from build123d import *

# Parameters (mm, degrees)
SKETCH_1_W                = 130
SKETCH_1_H                = 64
EXTRUDE_1_DEPTH           = 125
SKETCH_2_W                = 55.4
SKETCH_2_H                = 114
CUT_EXTRUDE_1_DEPTH       = 47
SKETCH_3_W                = 45.4
SKETCH_3_H                = 86
CUT_EXTRUDE_2_DEPTH       = 78
SKETCH_4_W                = 24.038907643
SKETCH_4_H                = 40
CUT_EXTRUDE_3_DEPTH       = 40
SKETCH_5_W                = 4.3
SKETCH_5_H                = 25
CUT_EXTRUDE_4_DEPTH       = 25
SKETCH_6_W                = 10
SKETCH_6_H                = 40
CUT_EXTRUDE_5_DEPTH       = 35
SKETCH_9_W                = 5
SKETCH_9_H                = 125
CUT_EXTRUDE_8_DEPTH       = 155.744951452
SKETCH_10_W               = 20
SKETCH_10_H               = 150
EXTRUDE_2_DEPTH           = 5
SKETCH_11_R               = 2.5
CUT_EXTRUDE_9_DEPTH       = 159.941026799
FILLET_1_R                = 3
SKETCH_12_W               = 32
SKETCH_12_H               = 30
CUT_EXTRUDE_10_DEPTH      = 161.864073055
SKETCH_13_W               = 45
SKETCH_13_H               = 50
CUT_EXTRUDE_11_DEPTH      = 30
FILLET_5_R                = 5
SKETCH_14_W               = 32
SKETCH_14_H               = 150
CUT_EXTRUDE_12_DEPTH      = 185.946613919
SKETCH_16_W               = 14.899109585
SKETCH_16_H               = 40
CUT_EXTRUDE_14_DEPTH      = 40
CUT_EXTRUDE_15_DEPTH      = 143.707007536
CUT_EXTRUDE_15_DEPTH_BACK = 143.707007536
SKETCH_17_W               = 30
SKETCH_17_H               = 95
SKETCH_18_W               = 20
SKETCH_18_H               = 6
CUT_EXTRUDE_16_DEPTH      = 150.244765402
SKETCH_20_W               = 47
SKETCH_20_H               = 10
EXTRUDE_3_DEPTH           = 10
SKETCH_21_R               = 1.75
CUT_EXTRUDE_17_DEPTH      = 141.388745988
SKETCH_23_W               = 42
SKETCH_23_H               = 27.7
CUT_EXTRUDE_19_DEPTH      = 138.927517197
EXTRUDE_4_DEPTH           = 27.7
SKETCH_25_W               = 48
SKETCH_25_H               = 23
EXTRUDE_5_DEPTH           = 4.3
FILLET_6_R                = 5
FILLET_8_R                = 5
CUT_EXTRUDE_23_DEPTH      = 10
SKETCH_31_R               = 1.55
CUT_EXTRUDE_24_DEPTH      = 138.669895039
FILLET_9_R                = 5
FILLET_10_R               = 5
FILLET_11_R               = 5


with BuildPart() as part:
    # 草图1 → 凸台-拉伸1 (new body)
    with BuildSketch(Plane(origin=(0, 0, 0), x_dir=(1, 0, 0), z_dir=(0, 1, 0))):
        Rectangle(SKETCH_1_W, SKETCH_1_H)
    extrude(amount=EXTRUDE_1_DEPTH)

    # 草图2 → 切除-拉伸1 (cut)
    with BuildSketch(Plane(origin=(65, 0, 0), x_dir=(0, 0, -1), z_dir=(1, 0, 0))):
        with Locations((0, 62)):
            Rectangle(SKETCH_2_W, SKETCH_2_H)
    extrude(amount=-CUT_EXTRUDE_1_DEPTH, mode=Mode.SUBTRACT)

    # 草图3 → 切除-拉伸2 (cut)
    with BuildSketch(Plane(origin=(18, 0, 0), x_dir=(0, 0, -1), z_dir=(1, 0, 0))):
        with Locations((0, 48)):
            Rectangle(SKETCH_3_W, SKETCH_3_H)
    extrude(amount=-CUT_EXTRUDE_2_DEPTH, mode=Mode.SUBTRACT)

    # 草图4 → 切除-拉伸3 (cut)
    with BuildSketch(Plane(origin=(65, 0, 0), x_dir=(0, 0, -1), z_dir=(1, 0, 0))):
        with Locations((26.569318974, 55)):
            Rectangle(SKETCH_4_W, SKETCH_4_H)
    extrude(amount=-CUT_EXTRUDE_3_DEPTH, mode=Mode.SUBTRACT)

    # 草图5 → 切除-拉伸4 (cut)
    with BuildSketch(Plane(origin=(65, 0, 0), x_dir=(0, 0, -1), z_dir=(1, 0, 0))):
        with Locations((29.85, 87.5)):
            Rectangle(SKETCH_5_W, SKETCH_5_H)
    extrude(amount=-CUT_EXTRUDE_4_DEPTH, mode=Mode.SUBTRACT)

    # 草图6 → 切除-拉伸5 (cut)
    with BuildSketch(Plane(origin=(0, 125, 0), x_dir=(1, 0, 0), z_dir=(0, 1, 0))):
        with Locations((45, 0)):
            Rectangle(SKETCH_6_W, SKETCH_6_H)
    extrude(amount=-CUT_EXTRUDE_5_DEPTH, mode=Mode.SUBTRACT)

    # 草图9 → 切除-拉伸8 (cut, through all)
    with BuildSketch(Plane.XY.offset(32)):
        with Locations((62.5, 62.5)):
            Rectangle(SKETCH_9_W, SKETCH_9_H)
    extrude(amount=-CUT_EXTRUDE_8_DEPTH, mode=Mode.SUBTRACT)

    # 草图10 → 凸台-拉伸2 (add)
    with BuildSketch(Plane(origin=(0, 0, -32), x_dir=(-1, 0, 0), z_dir=(0, 0, -1))):
        with Locations((15, 57.5)):
            Rectangle(SKETCH_10_W, SKETCH_10_H)
    extrude(amount=-EXTRUDE_2_DEPTH)

    # 草图11 → 切除-拉伸9 (cut, through all)
    with BuildSketch(Plane.XY.offset(-27)):
        with Locations((-15, -12)):
            Circle(SKETCH_11_R)
        with Locations((-15, 137)):
            Circle(SKETCH_11_R)
    extrude(amount=-CUT_EXTRUDE_9_DEPTH, mode=Mode.SUBTRACT)

    # 圆角1
    fillet_1_edges = [part.edges().sort_by_distance(p)[0] for p in [
        (-15, 0, -27),
        (-5, 0, -29.5),
        (-25, 0, -29.5),
        (-25, 132.5, -29.5),
        (-25, 125, -29.5),
        (-5, 125, -29.5),
        (-15, 125, -27),
        (-25, -17.5, -29.5),
        (-5, -17.5, -29.5),
        (-5, 132.5, -29.5),
    ]]
    fillet(fillet_1_edges, radius=FILLET_1_R)

    # 草图12 → 切除-拉伸10 (cut, through all)
    with BuildSketch(Plane.XY.offset(32)):
        with Locations((-49, 110)):
            Rectangle(SKETCH_12_W, SKETCH_12_H)
    extrude(amount=-CUT_EXTRUDE_10_DEPTH, mode=Mode.SUBTRACT)

    # 草图13 → 切除-拉伸11 (cut)
    with BuildSketch(Plane(origin=(0, 125, 0), x_dir=(1, 0, 0), z_dir=(0, 1, 0))):
        with Locations((-10.5, -7)):
            Rectangle(SKETCH_13_W, SKETCH_13_H)
    extrude(amount=-CUT_EXTRUDE_11_DEPTH, mode=Mode.SUBTRACT)

    # 圆角5
    fillet_5_edges = [part.edges().sort_by_distance(p)[0] for p in [
        (-33, 110, -18),
        (12, 110, -18),
    ]]
    fillet(fillet_5_edges, radius=FILLET_5_R)

    # 草图14 → 切除-拉伸12 (cut, through all)
    with BuildSketch(Plane.ZY.offset(65)):
        with Locations((-16, 57.5)):
            Rectangle(SKETCH_14_W, SKETCH_14_H)
    extrude(amount=-CUT_EXTRUDE_12_DEPTH, mode=Mode.SUBTRACT)

    # 草图16 → 切除-拉伸14 (cut)
    with BuildSketch(Plane(origin=(60, 0, 0), x_dir=(0, 0, -1), z_dir=(1, 0, 0))):
        with Locations((-29.056746571, 55)):
            Rectangle(SKETCH_16_W, SKETCH_16_H)
    extrude(amount=-CUT_EXTRUDE_14_DEPTH, mode=Mode.SUBTRACT)

    # 草图17 → 切除-拉伸15 (cut, two sides: drawn at the far end of the back side and taken through both)
    with BuildSketch(Plane(origin=(0, 0, 22.7), x_dir=(-1, 0, 0), z_dir=(0, 0, -1)).offset(-CUT_EXTRUDE_15_DEPTH_BACK)):
        with Locations((50, 47.5)):
            Rectangle(SKETCH_17_W, SKETCH_17_H)
    extrude(amount=CUT_EXTRUDE_15_DEPTH + CUT_EXTRUDE_15_DEPTH_BACK, mode=Mode.SUBTRACT)

    # 草图18 → 切除-拉伸16 (cut, through all)
    with BuildSketch(Plane(origin=(40, 0, 0), x_dir=(0, 0, -1), z_dir=(1, 0, 0))):
        with Locations((-10, 122)):
            Rectangle(SKETCH_18_W, SKETCH_18_H)
    extrude(amount=CUT_EXTRUDE_16_DEPTH, mode=Mode.SUBTRACT)

    # 草图20 → 凸台-拉伸3 (add)
    with BuildSketch(Plane.XY.offset(32)):
        with Locations((-11.5, -5)):
            Rectangle(SKETCH_20_W, SKETCH_20_H)
        with Locations((-11.5, 100)):
            Rectangle(SKETCH_20_W, SKETCH_20_H)
    extrude(amount=-EXTRUDE_3_DEPTH)

    # 草图21 → 切除-拉伸17 (cut, through all)
    with BuildSketch(Plane(origin=(0, 0, 22), x_dir=(-1, 0, 0), z_dir=(0, 0, -1))):
        with Locations(Location((25, -5, 0), (0, 0, 180))):
            Circle(SKETCH_21_R)
        with Locations(Location((5, -5, 0), (0, 0, 180))):
            Circle(SKETCH_21_R)
        with Locations((5, 100)):
            Circle(SKETCH_21_R)
        with Locations((25, 100)):
            Circle(SKETCH_21_R)
    extrude(amount=-CUT_EXTRUDE_17_DEPTH, mode=Mode.SUBTRACT)

    # 草图23 → 切除-拉伸19 (cut, through all)
    with BuildSketch(Plane(origin=(0, 5, 0), x_dir=(1, 0, 0), z_dir=(0, 1, 0))):
        with Locations((39, -13.85)):
            Rectangle(SKETCH_23_W, SKETCH_23_H)
    extrude(amount=-CUT_EXTRUDE_19_DEPTH, mode=Mode.SUBTRACT)

    # 草图24 → 凸台-拉伸4 (add)
    with BuildSketch(Plane(origin=(0, 0, 0), x_dir=(-1, 0, 0), z_dir=(0, 0, -1))):
        Polygon((-18, 0), (-18, -17), (-60, -17), (-60, -23), (-12, -23), (-12, 0), align=None)
    extrude(amount=-EXTRUDE_4_DEPTH)

    # 草图25 → 凸台-拉伸5 (add)
    with BuildSketch(Plane.XY.offset(32)):
        with Locations((36, -11.5)):
            Rectangle(SKETCH_25_W, SKETCH_25_H)
    extrude(amount=-EXTRUDE_5_DEPTH)

    # 圆角6
    fillet_6_edges = [part.edges().sort_by_distance(p)[0] for p in [
        (-35, 105, 27),
        (12, 105, 27),
        (-35, -10, 27),
        (12, -10, 27),
    ]]
    fillet(fillet_6_edges, radius=FILLET_6_R)

    # 圆角8
    fillet_8_edges = [part.edges().sort_by_distance(p)[0] for p in [
        (12, 95, 11),
    ]]
    fillet(fillet_8_edges, radius=FILLET_8_R)

    # 草图30 → 切除-拉伸23 (cut)
    with BuildSketch(Plane(origin=(0, 0, 22), x_dir=(-1, 0, 0), z_dir=(0, 0, -1))):
        with BuildLine():
            Line((-7, 105), (-3, 105))
            Line((-3, 105), (-3, 95))
            Line((-3, 95), (-7, 95))
            ThreePointArc((-7, 95), (-10.535533906, 96.464466094), (-12, 100))
            Line((-12, 100), (-12, 110))
            ThreePointArc((-12, 110), (-10.535533906, 106.464466094), (-7, 105))
        make_face()
        with BuildLine():
            Line((-7, -10), (-3, -10))
            Line((-3, -10), (-3, 0))
            Line((-3, 0), (-12, 0))
            Line((-12, 0), (-12, -15))
            ThreePointArc((-12, -15), (-10.535533906, -11.464466094), (-7, -10))
        make_face()
    extrude(amount=-CUT_EXTRUDE_23_DEPTH, mode=Mode.SUBTRACT)

    # 草图31 → 切除-拉伸24 (cut, through all)
    with BuildSketch(Plane.ZY.offset(-12)):
        with Locations(Location((23.7, 113.3, 0), (0, 0, 270))):
            Circle(SKETCH_31_R)
        with Locations(Location((23.7, -12.3, 0), (0, 0, 270))):
            Circle(SKETCH_31_R)
    extrude(amount=-CUT_EXTRUDE_24_DEPTH, mode=Mode.SUBTRACT)

    # 圆角9
    fillet_9_edges = [part.edges().sort_by_distance(p)[0] for p in [
        (12, 0, 16),
    ]]
    fillet(fillet_9_edges, radius=FILLET_9_R)

    # 圆角10
    fillet_10_edges = [part.edges().sort_by_distance(p)[0] for p in [
        (3, -10, 27),
    ]]
    fillet(fillet_10_edges, radius=FILLET_10_R)

    # 圆角11
    fillet_11_edges = [part.edges().sort_by_distance(p)[0] for p in [
        (3, 105, 27),
    ]]
    fillet(fillet_11_edges, radius=FILLET_11_R)


solid = part.part
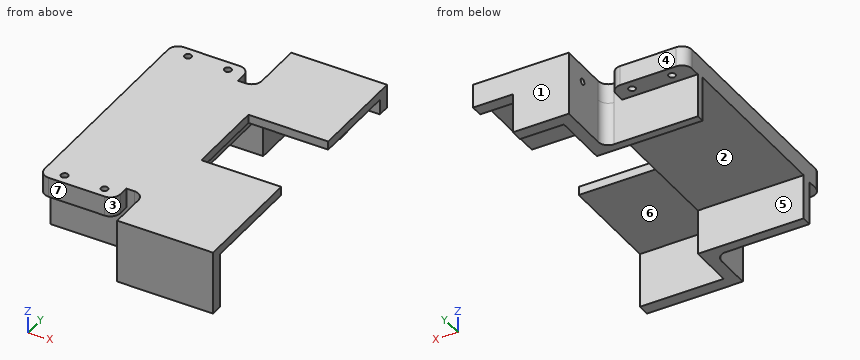
Work out the finished part from the listing and answer in its coordinate system (mm). Face numbers are marked on the shaded views. A direction names the side the tool comes from. Coordinates: 2 decimals unless noted, no trailing zeros. Write each loop counter-clockwise with the first axis right and the second up, starting at its lowest first coordinate (ties: lowest second). Pieces come first, ordered by that corner, then holes. Notation, with made-up numbers: M 80,-35 L 84,-35 A13 ccw 84,-21 Z; hole C -3.5,23.5 d7. An arc over 180 degrees is marked long. Write item = value, one per line.
1. Flat-ended cylindrical pins translate along their axes: pin 1 (8 mm diameter, centred on x = 5.5, z = 17.5, fed in from +Y); pin 2 (1.3 mm diameter, centred on y = 57.5, z = 29.5, fed in from +X); pin 3 (14 mm diameter, centred on y = 75, z = 20.5, fed in from +X). Find the tip coordinate at first contact, or state that the pin passes through.
Solution:
pin_1 = 95.67
pin_2 = 20
pin_3 = 18
2. Determine the mould class of the marked faces 1, 2 and 3 for opening direction Y: released by +Y, released by -Y, zero draft, split by the parting line, or undercut.
Solution:
face_1 = released by +Y
face_2 = undercut
face_3 = released by -Y
3. The part is cut by section B-B (x = 46.5). Determine the outline of the cut face in (y, z).
Solution:
outline = M -23,0 L -17,0 L -17,27.7 L 35,27.7 L 35,32 L -23,32 Z; M 75,27.7 L 119,27.7 L 119,20 L 125,20 L 125,32 L 75,32 Z
4. Straight lines are drawn through the part: line 1 (X direction, y = 100, z = 24.5); line 2 (X direction, y = 100, z = 30.25); line 3 (Y direction, x = -25, z = 24). For each, find the intervals that lie inside material, in ascending order. Write a range as from..to.
Solution:
line_1 = -35..-26.75, -23.25..-6.75, -3.25..3, 12..18
line_2 = -35..-26.75, -23.25..-6.75, -3.25..3, 12..60
line_3 = -10..-6.75, -3.25..98.25, 101.75..105
5. The part is cut by section C-C (x = -5). Determine the outline of the cut face in (y, z).
Solution:
outline = M -10,22 L -6.75,22 L -6.75,32 L -10,32 Z; M -3.25,22 L 0,22 L 0,0 L 5,0 L 5,22.7 L 91,22.7 L 91,0 L 95,0 L 95,22 L 98.25,22 L 98.25,32 L -3.25,32 Z; M 101.75,22 L 105,22 L 105,32 L 101.75,32 Z
6. For the marked faces 4, 5, 6 and 7, determine the directions among +Z, -Z, +X, -X, +Y, -Y from which every point of the face is accessible in a straight line to the end or side of a thin tool.
Solution:
face_4 = +Z, -Z, -X, +Y
face_5 = -Z, +X, -X
face_6 = -Z, +X
face_7 = +Z, -Z, -X, -Y
7. The part is cut by section D-D (y = 113.3). Determine the outline of the cut face in (x, z), then the cut area to 3 significant figures.
Solution:
outline = M 12,0 L 18,0 L 18,22.15 L 12,22.15 Z; M 12,25.25 L 18,25.25 L 18,27.7 L 60,27.7 L 60,32 L 12,32 Z
area = 354 mm2
8. The part is cut by section A-A (z = 10). Determine the outline of the cut face in (x, y).
Solution:
outline = M -35,0 L 7,0 A5 cw 12,-5 L 12,-23 L 60,-23 L 60,-17 L 18,-17 L 18,5 L -35,5 Z; M -35,91 L 18,91 L 18,119 L 40,119 L 40,125 L 12,125 L 12,100 A5 cw 7,95 L -35,95 Z
